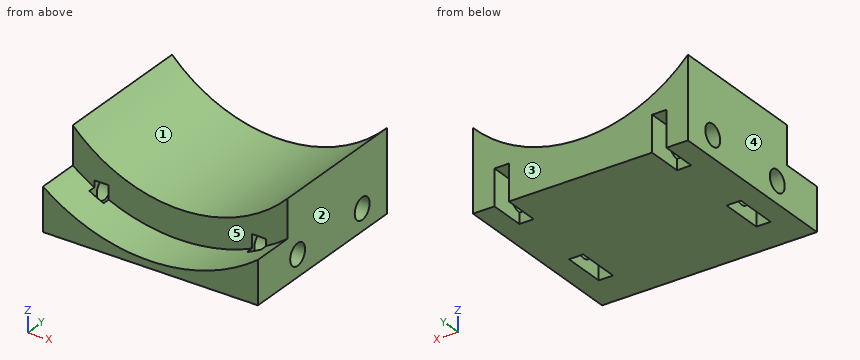
```python
from build123d import *

# Parameters (mm, degrees)
CYLINDER2795_R     = 1.5
CYLINDER2795_DEPTH = 64
CYLINDER2794_R     = 1.5
CYLINDER2794_DEPTH = 64
CYLINDER2793_R     = 38
CYLINDER2793_DEPTH = 30
BOX983_W           = 2
BOX983_H           = 6
BOX983_DEPTH       = 6
BOX984_W           = 2
BOX984_H           = 6
BOX984_DEPTH       = 6
BOX985_W           = 2
BOX985_H           = 6
BOX985_DEPTH       = 6
BOX986_W           = 2
BOX986_H           = 6
BOX986_DEPTH       = 6
BOX987_W           = 2
BOX987_H           = 6
BOX987_DEPTH       = 6
BOX989_W           = 2
BOX989_H           = 6
BOX989_DEPTH       = 6
TUBE139_R          = 21
TUBE139_R_2        = 2
TUBE139_DEPTH      = 64
TUBE140_R          = 25
TUBE140_R_2        = 2
TUBE140_DEPTH      = 26
BOX988_W           = 30
BOX988_H           = 64
BOX988_DEPTH       = 18
BOX982_W           = 30
BOX982_H           = 26
BOX982_DEPTH       = 18


with BuildPart() as obj1:
    # Cylinder2795 → Cylinder2795 (new body)
    with BuildSketch(Plane(origin=(-26, 12, 14), x_dir=(0, 0, -1), z_dir=(1, 0, 0))):
        Circle(CYLINDER2795_R)
    extrude(amount=CYLINDER2795_DEPTH)


with BuildPart() as compound1245:
    # Cylinder2794 → Cylinder2794 (new body)
    with BuildSketch(Plane(origin=(-26, -1, 14), x_dir=(0, 0, -1), z_dir=(1, 0, 0))):
        Circle(CYLINDER2794_R)
    extrude(amount=CYLINDER2794_DEPTH)

    # Compound1245: union obj1
    add(obj1.part)


with BuildPart() as obj2:
    # Cylinder2793 → Cylinder2793 (new body)
    with BuildSketch(Plane.XY):
        Circle(CYLINDER2793_R)
    extrude(amount=CYLINDER2793_DEPTH)


with BuildPart() as krychle982:
    # Box983 → Box983 (new body)
    with BuildSketch(Plane(origin=(-12, -4, 10), x_dir=(1, 0, 0), z_dir=(0, 0, 1))):
        with Locations((1, 3)):
            Rectangle(BOX983_W, BOX983_H)
    extrude(amount=BOX983_DEPTH)


with BuildPart() as krychle983:
    # Box984 → Box984 (new body)
    with BuildSketch(Plane(origin=(10, 26, 10), x_dir=(1, 0, 0), z_dir=(0, 0, 1))):
        with Locations((1, 3)):
            Rectangle(BOX984_W, BOX984_H)
    extrude(amount=BOX984_DEPTH)


with BuildPart() as krychle984:
    # Box985 → Box985 (new body)
    with BuildSketch(Plane(origin=(-12, 26, 10), x_dir=(1, 0, 0), z_dir=(0, 0, 1))):
        with Locations((1, 3)):
            Rectangle(BOX985_W, BOX985_H)
    extrude(amount=BOX985_DEPTH)


with BuildPart() as krychle985:
    # Box986 → Box986 (new body)
    with BuildSketch(Plane(origin=(10, 12, 10), x_dir=(1, 0, 0), z_dir=(0, 0, 1))):
        with Locations((1, 3)):
            Rectangle(BOX986_W, BOX986_H)
    extrude(amount=BOX986_DEPTH)


with BuildPart() as krychle986:
    # Box987 → Box987 (new body)
    with BuildSketch(Plane(origin=(-12, 12, 10), x_dir=(1, 0, 0), z_dir=(0, 0, 1))):
        with Locations((1, 3)):
            Rectangle(BOX987_W, BOX987_H)
    extrude(amount=BOX987_DEPTH)


with BuildPart() as compound1244:
    # Box989 → Box989 (new body)
    with BuildSketch(Plane(origin=(10, -4, 10), x_dir=(1, 0, 0), z_dir=(0, 0, 1))):
        with Locations((1, 3)):
            Rectangle(BOX989_W, BOX989_H)
    extrude(amount=BOX989_DEPTH)

    # Compound1244: union Krychle982, Krychle983, Krychle984, Krychle985, Krychle986
    add(krychle982.part)
    add(krychle983.part)
    add(krychle984.part)
    add(krychle985.part)
    add(krychle986.part)


with BuildPart() as tube139:
    # Tube139 → Tube139 (new body)
    with BuildSketch(Plane(origin=(0, 61, 37), x_dir=(1, 0, 0), z_dir=(0, -1, 0))):
        Circle(TUBE139_R)
        Circle(TUBE139_R_2, mode=Mode.SUBTRACT)
    extrude(amount=TUBE139_DEPTH)


with BuildPart() as tube140:
    # Tube140 → Tube140 (new body)
    with BuildSketch(Plane(origin=(0, -3, 37), x_dir=(1, 0, 0), z_dir=(0, -1, 0))):
        Circle(TUBE140_R)
        Circle(TUBE140_R_2, mode=Mode.SUBTRACT)
    extrude(amount=TUBE140_DEPTH)


with BuildPart() as common009:
    # Box988 → Box988 (new body)
    with BuildSketch(Plane(origin=(-15, -17, 11), x_dir=(1, 0, 0), z_dir=(0, 0, 1))):
        with Locations((15, 32)):
            Rectangle(BOX988_W, BOX988_H)
    extrude(amount=BOX988_DEPTH)

    # Cut1053: cut Tube140
    add(tube140.part, mode=Mode.SUBTRACT)

    # Cut1054: cut Tube139
    add(tube139.part, mode=Mode.SUBTRACT)

    # Cut1055: cut Compound1244
    add(compound1244.part, mode=Mode.SUBTRACT)

    # Common009: intersect obj2
    add(obj2.part, mode=Mode.INTERSECT)


with BuildPart() as cut1056:
    # Box982 → Box982 (new body)
    with BuildSketch(Plane(origin=(-15, -9, 11), x_dir=(1, 0, 0), z_dir=(0, 0, 1))):
        with Locations((15, 13)):
            Rectangle(BOX982_W, BOX982_H)
    extrude(amount=BOX982_DEPTH)

    # Common010: intersect Common009
    add(common009.part, mode=Mode.INTERSECT)

    # Cut1056: cut Compound1245
    add(compound1245.part, mode=Mode.SUBTRACT)


solid = cut1056.part
```
The listing builds one solid part. Answer for the finished solid, in the listing's coordinates (mm). Face numbers are marked on the shaded views. A direction names the side the tool comes from. Coordinates: 2 decimals unless noted, no trailing zeros. Loops run counter-clockwise (first coordinate to the right, second up) from the corner with the lowest first, then second, coordinate; pieces in that order, holes last. Notation, with made-up numbers: (86.25, 21.5) - (116.25, 21.5) arc R17 ccw to (116.25, 36.5) - close; hole circle Ø10 at (85, 1). An arc over 180 degrees is marked (long way). Use a Markdown table: item, result. Add a question column.
1) For the marked faces 4 and 5, determine the directions among +Z, -Z, +X, -X, +Y, -Y from which every point of the face is accessible in a straight line to the end or side of a thin tool.
2) The part is cut by section D-D, the plane x = 8. Give the vertices of the cut face in (y, z).
3) Given pin 1 (0.6 mm diameter, centred on x = -10.5, y = -1, fed in from -Z); pin 2 (0.8 mm diameter, centred on x = 11.5, z = 12, fed in from +Y); pin 3 (5 mm diameter, centred on y = -1, z = 14, fed in from +X); pin 4 (6 mm diameter, centred on x = -0.5, y = 8.5, fed in from +Z), each flat-ended and moving along its own axis, determine where each tip first touches the part or whether it passes through.
4) The part is cut by section C-C, the plane x = -11. Give the vertices of the cut face in (y, z), and give its area (3 significant figures).
5) The part is cut by section A-A, the plane y = -1. Give the vertices of the cut face in (x, z), and give its area (3 significant figures).
6) Find the intervals of material crossed by line 1 (Y direction, x = -13, z = 14); line 2 (Y direction, x = 4, z = 14); line 3 (X direction, y = 0.5, z = 12.75), in increasing order.
7) The mould has two halves that part along X. Classify the marked faces 1, 2 and 3: released by +X, released by -X, zero draft, split by the parting line, or undercut.
8) The part is cut by section B-B, the plane z = 17.5. Give the vertices of the cut face in (x, y).
Here are the results:
| question | item | result |
|---|---|---|
| 1 | face 4 | +Z, -Z, -X, +Y, -Y |
| 1 | face 5 | +Z, -Y |
| 2 | outline | (-9, 11) - (17, 11) - (17, 17.58) - (-3, 17.58) - (-3, 13.31) - (-9, 13.31) - close; hole circle Ø3 at (-1, 14); hole circle Ø3 at (12, 14) |
| 3 | pin 1 | stops at z = 16 |
| 3 | pin 2 | stops at y = 12 |
| 3 | pin 3 | stops at x = 15 |
| 3 | pin 4 | stops at z = 16.29 |
| 4 | outline | (-9, 11) - (-4, 11) - (-4, 14.55) - (-9, 14.55) - close; (-3, 16) - (2, 16) - (2, 11) - (12, 11) - (12, 12.5) arc R1.5 cw to (12, 15.5) - (12, 16) - (17, 16) - (17, 19.11) - (-3, 19.11) - close |
| 4 | area | 126 mm^2 |
| 5 | outline | (-15, 11) - (-12, 11) - (-12, 12.5) - (-15, 12.5) - close; (-15, 15.5) - (-12, 15.5) - (-12, 16) - (-10, 16) - (-10, 15.5) - (10, 15.5) - (10, 16) - (12, 16) - (12, 15.5) - (15, 15.5) - (15, 22.3) arc R21 cw to (-15, 22.3) - close; (-10, 11) - (10, 11) - (10, 12.5) - (-10, 12.5) - close; (12, 11) - (15, 11) - (15, 12.5) - (12, 12.5) - close |
| 5 | area | 111 mm^2 |
| 6 | line 1 | y = -9 to -2.5, 0.5 to 10.5, 13.5 to 17 |
| 6 | line 2 | y = -3 to -2.5, 0.5 to 10.5, 13.5 to 17 |
| 6 | line 3 | x = -15 to -12, -10 to 10, 12 to 15 |
| 7 | face 1 | undercut |
| 7 | face 2 | released by +X |
| 7 | face 3 | zero draft |
| 8 | outline | (-15, -3) - (-7.79, -3) - (-7.79, 17) - (-15, 17) - close; (7.79, -3) - (15, -3) - (15, 17) - (7.79, 17) - close |
